The figure shows three views and two pictorial views of one solid part (mm, origin at its lowest corner). Answer the questions. A direction names the side the tool comes from. Give positions to 0.01 mm unless a question says otherwise; leave off trailing zeros. Write each loop counter-clockwise with the first axis right and the second up, starting at its lowest first coordinate (ties: lowest second). Pieces come first, ordered by that corner, then holes. Notation, with made-up numbers: (11.5, 24) -> (62.5, 24) arc R5 ccw to (62.5, 33) -> close; hole circle Ø5 at (11.5, 82). An arc over 180 degrees is marked (long way). Use a Markdown table: item, result.
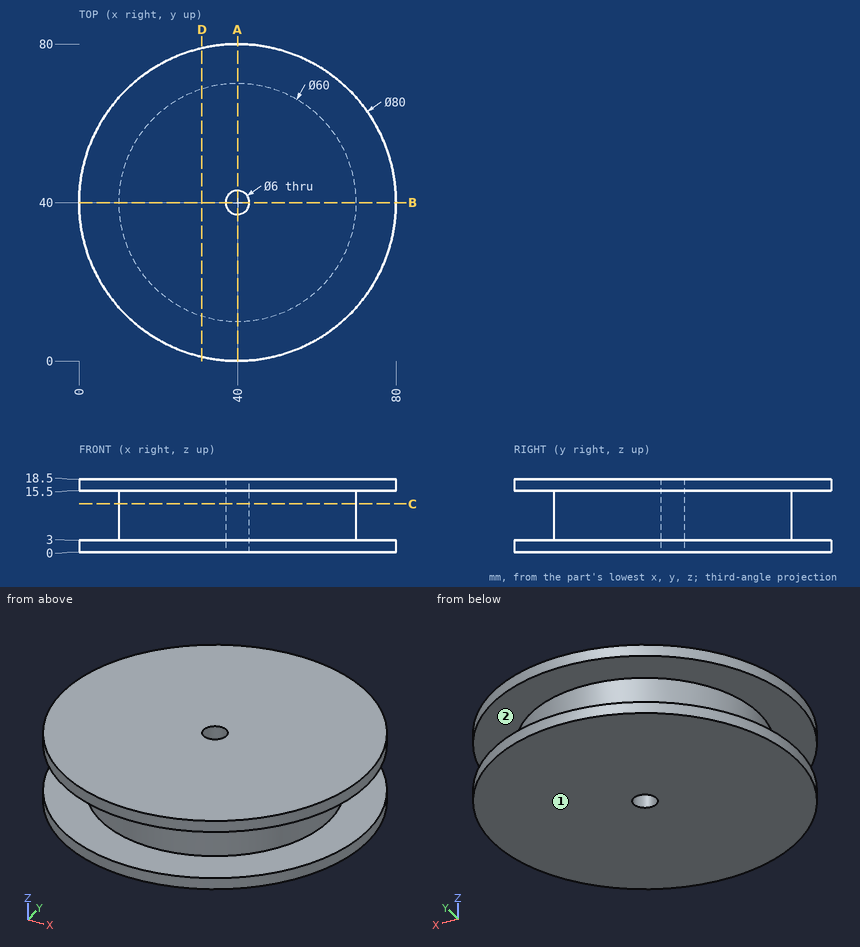
Item 1: A cutting plane is placed at D-D (x = 31). Give the vertices of the cut face in (y, z).
Return value:
| item | result |
|---|---|
| outline | (1.03, 0) -> (78.97, 0) -> (78.97, 3) -> (68.62, 3) -> (68.62, 15.5) -> (78.97, 15.5) -> (78.97, 18.5) -> (1.03, 18.5) -> (1.03, 15.5) -> (11.38, 15.5) -> (11.38, 3) -> (1.03, 3) -> close |
Item 2: A tool of negligible diameter and unlimited length cuts with its end or side. For the marked faces 1 and 2, from which of +Z, -Z, +X, -X, +Y, -Y can it reach the whole face along a straight path? Write none if from no direction.
Return value:
| item | result |
|---|---|
| face 1 | -Z, +X, -X, +Y, -Y |
| face 2 | none |
Item 3: A cutting plane is placed at C-C (z = 12.25). Give the vertices of the cut face in (x, y).
Return value:
| item | result |
|---|---|
| outline | circle Ø60 at (40, 40); hole circle Ø6 at (40, 40) |
Item 4: Straight lines are drawn through the part: line 1 along Z through (x, y) = (67.5, 60); line 2 along Y through (x, z) = (40, 11.75); line 3 along Y through (x, z) = (49, 4.75). For each, find the intervals that lie inside material, in ascending order. Write a range as [from, to].
Return value:
| item | result |
|---|---|
| line 1 | [0, 3], [15.5, 18.5] |
| line 2 | [10, 37], [43, 70] |
| line 3 | [11.38, 68.62] |
Item 5: Each of these flat-tipped pins is pushed along its axis until it touches: P1, Ø3, axis at x = 16, z = 12, coming from the +Y side; P2, Ø5.5, axis at x = 40, y = 40, coming from the -Z side; P3, Ø10, axis at y = 51, z = 4.5, coming from the -X side. Where does it stop, or does it pass through?
Return value:
| item | result |
|---|---|
| P1 | y = 59.84 |
| P2 | through |
| P3 | x = 0.49 |
Item 6: A cutting plane is placed at A-A (x = 40). Give the vertices of the cut face in (y, z).
Return value:
| item | result |
|---|---|
| outline | (0, 0) -> (37, 0) -> (37, 18.5) -> (0, 18.5) -> (0, 15.5) -> (10, 15.5) -> (10, 3) -> (0, 3) -> close; (43, 0) -> (80, 0) -> (80, 3) -> (70, 3) -> (70, 15.5) -> (80, 15.5) -> (80, 18.5) -> (43, 18.5) -> close |
